For this review, use the dimensioned drawing (mm, ordinates from the lowest corner) and the shaded views. Coordinates: 2 decimals unless noted, no trailing zeros. Order: outer loops, then holes, each group sorted by start corner. A loop starts at its lowest first (then second) coordinate and runs counter-clockwise, first axis right, second up. Notation, with made-up numbers: (33, 62) -> (65, 62) arc R30 cw to (65, 100) -> close; hole circle Ø1 at (31.25, 80). An arc over 180 degrees is marked (long way). Return JSON: item names as keys, results as strings. Group by question number.
Item 1: Draft analysis for pull direction X (two halves, no side actions). For the marked faces 1 and 2, state which applies: +X half, -X half, draft (parallel to the pull), parting line (faces both ways), or undercut.
Item 2: Take a section at C-C (z = 1.55). Write out the cut boundary in (x, y).
Item 3: Take a section at B-B (y = 5.08). Write out the cut boundary in (x, z), then the cut area to 3 significant figures.
Item 4: Take a section at A-A (x = 31.75). Write out the cut boundary in (y, z).
Item 5: For line 1 along Y through (x, z) = (31.75, 1.4); line 2 along Y through (x, z) = (23, 2.4); line 3 along X through (y, z) = (4.25, 1.9), list the stretches that pass through material, from the lowest coordinate up.
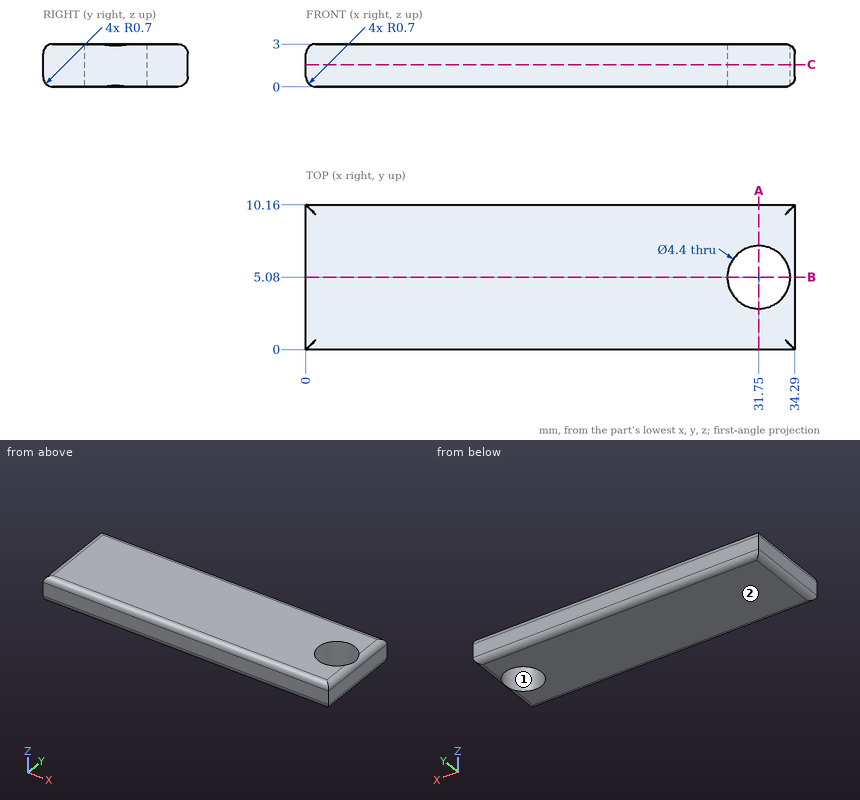
Findings below:
{
 "1": {"face 1": "undercut", "face 2": "draft"},
 "2": {"outline": "(0, 0) -> (34.29, 0) -> (34.29, 10.16) -> (0, 10.16) -> close; hole circle Ø4.4 at (31.75, 5.08)"},
 "3": {"outline": "(0, 0.7) arc R0.7 ccw to (0.7, 0) -> (29.55, 0) -> (29.55, 3) -> (0.7, 3) arc R0.7 ccw to (0, 2.3) -> close; (33.95, 0.1) arc R0.7 ccw to (34.29, 0.7) -> (34.29, 2.3) arc R0.7 ccw to (33.95, 2.9) -> close", "area": "89.3 mm2"},
 "4": {"outline": "(0, 0.7) arc R0.7 ccw to (0.7, 0) -> (2.88, 0) -> (2.88, 3) -> (0.7, 3) arc R0.7 ccw to (0, 2.3) -> close; (7.28, 0) -> (9.46, 0) arc R0.7 ccw to (10.16, 0.7) -> (10.16, 2.3) arc R0.7 ccw to (9.46, 3) -> (7.28, 3) -> close"},
 "5": {"line 1": "y = 0 to 2.88, 7.28 to 10.16", "line 2": "y = 0.01 to 10.15", "line 3": "x = 0 to 29.71, 33.79 to 34.29"}
}
